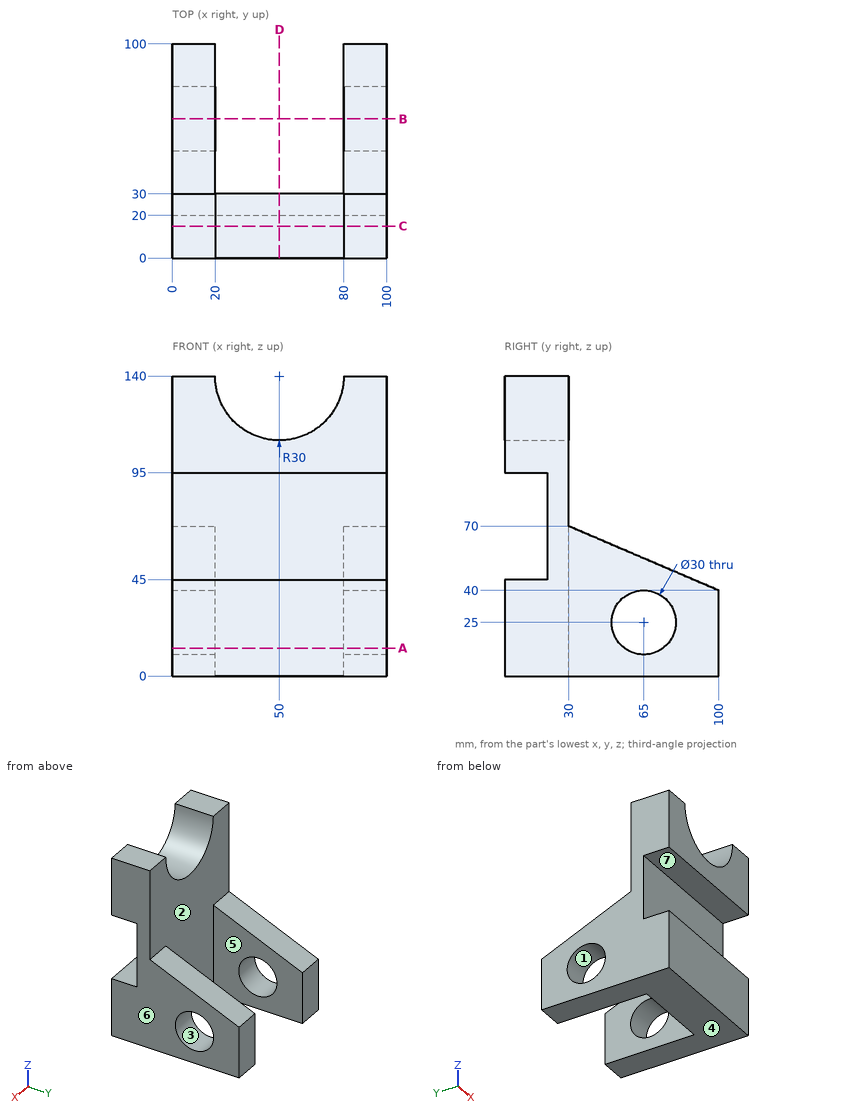
Input: dimensioned drawing with shaded views. Units: mm. Origin: part minimum x, y, z. A direction names the side the tool comes from. Give positions to 0.01 mm unless a question says otherwise; leave off trailing zeros. Write each loop counter-clockwise with the first axis right and the second up, starting at its lowest first coordinate (ties: lowest second). Pieces come first, ordered by that corner, then holes.
Q1. Section C-C, the plane y = 15. Output: boundary loops of the cut face in (x, z).
Q2. First-contact query: P1, Ø16, axis at x = 31.5, y = 8, coming from the +Z side; P2, Ø1, axis at x = 15.5, z = 56.5, coming from the +Y side; P3, Ø1, axis at x = 21, z = 72, coming from the +Y side. Flat tips, straight axial feed; report the tip coordinate or a pass-through.
Q3. Material intervals for probe 1 along X at (y, z) = (85.5, 32); probe 2 along Y at (x, z) = (88, 25); probe 3 along Y at (x, z) = (56.5, 40.5), sorted ascending.
Q4. Pull-direction query (Y, two-part tool) for the marked faces 1, 2, 3 and 4; classes: pulls with the +Y half, pulls with the -Y half, needs draft (parallel to the pull), parting line crosses it, or undercut.
Q5. Section B-B, the plane y = 65. Output: boundary loops of the cut face in (x, z), plus the area to 3 significant figures.
Q6. Section D-D, the plane x = 50. Output: boundary loops of the cut face in (y, z), plus the area to 3 significant figures.
Q7. Section A-A, the plane z = 13. Output: boundary loops of the cut face in (x, y).
Q8. Set-up query: the marked faces 5, 6 and 7. Return all of +Z, -Z, +X, -X, +Y, -Y with unobstructed straight access to the full face (end or side cutting, diameter ignored); none if empty.
Filled in:
1. outline: (0, 0) - (100, 0) - (100, 45) - (0, 45) - close; (0, 95) - (100, 95) - (100, 140) - (80, 140) arc R30 cw to (20, 140) - (0, 140) - close
2. P1: stops at z = 125.94
2. P2: stops at y = 62.67
2. P3: stops at y = 30
3. probe 1: x = 0 to 20, 80 to 100
3. probe 2: y = 0 to 50, 80 to 100
3. probe 3: y = 0 to 30
4. face 1: undercut
4. face 2: pulls with the +Y half
4. face 3: undercut
4. face 4: needs draft
5. outline: (0, 0) - (20, 0) - (20, 10) - (0, 10) - close; (0, 40) - (20, 40) - (20, 55) - (0, 55) - close; (80, 0) - (100, 0) - (100, 10) - (80, 10) - close; (80, 40) - (100, 40) - (100, 55) - (80, 55) - close
5. area: 1,000 mm2
6. outline: (0, 0) - (30, 0) - (30, 110) - (0, 110) - (0, 95) - (20, 95) - (20, 45) - (0, 45) - close
6. area: 2,300 mm2
7. outline: (0, 0) - (100, 0) - (100, 56) - (80, 56) - (80, 30) - (20, 30) - (20, 56) - (0, 56) - close; (0, 74) - (20, 74) - (20, 100) - (0, 100) - close; (80, 74) - (100, 74) - (100, 100) - (80, 100) - close
8. face 5: +Z, -Z, +Y
8. face 6: +Z, -Z, +X, +Y, -Y
8. face 7: +X, -X, -Y
